Check sheet for the drawn part. Datum: minimum x, y, z corner. Units: mm. A direction names the side the tool comes from. Round coordinates to 2 decimals unless told otherwise and drop trailing zeros. Write each loop counter-clockwise with the first axis right and the second up, starting at its lowest first coordinate (ties: lowest second). Pieces come first, ordered by that corner, then holes. Notation, with made-up numbers: M 54,44.25 L 108,44.25 A7 cw 108,56.25 Z; hole C 13.25,14 d5. An arc over 180 degrees is marked long. One line per item, written item: value. Start each with the question number.
1. Depth check by flat-ended pin: P1, Ø5, axis at x = 35.5, y = 66.5, coming from the +Z side; P2, Ø3, axis at x = 37, y = 32.5, coming from the -Z side; P3, Ø8, axis at x = 83, z = 69, coming from the +Y side. Enter the tip coordinate at first touch or a pass-through.
2. Section check B-B (y = 69.85). Record the boundary of the cut face in (x, z), and give its area (3 significant figures).
3. Section check A-A (x = 50.8). Record the boundary of the cut face in (y, z), and give its area (3 significant figures).
4. Access from +Z, -Z, +X, -X, +Y, -Y to the whole of each face (thin tool, end or side, straight path). Record for the marked faces 1 and 2.
5. Section check D-D (z = 50.8). Record the boundary of the cut face in (x, y).
6. Release check for a two-part mould opening along Z. For the marked faces 3, 4 and 5 record: pulls with the +Z half, pulls with the -Z half, needs draft (parallel to the pull), parting line crosses it, or undercut.
7. Scan lines: probe 1 along Y at (x, z) = (50.8, 92.25); probe 2 along X at (y, z) = (69, 5); probe 3 along X at (y, z) = (69, 97). Record each from-to range of solid material in increasing order. Write a range as [from, to].
8. Section check C-C (y = 57). Record the boundary of the cut face in (x, z).
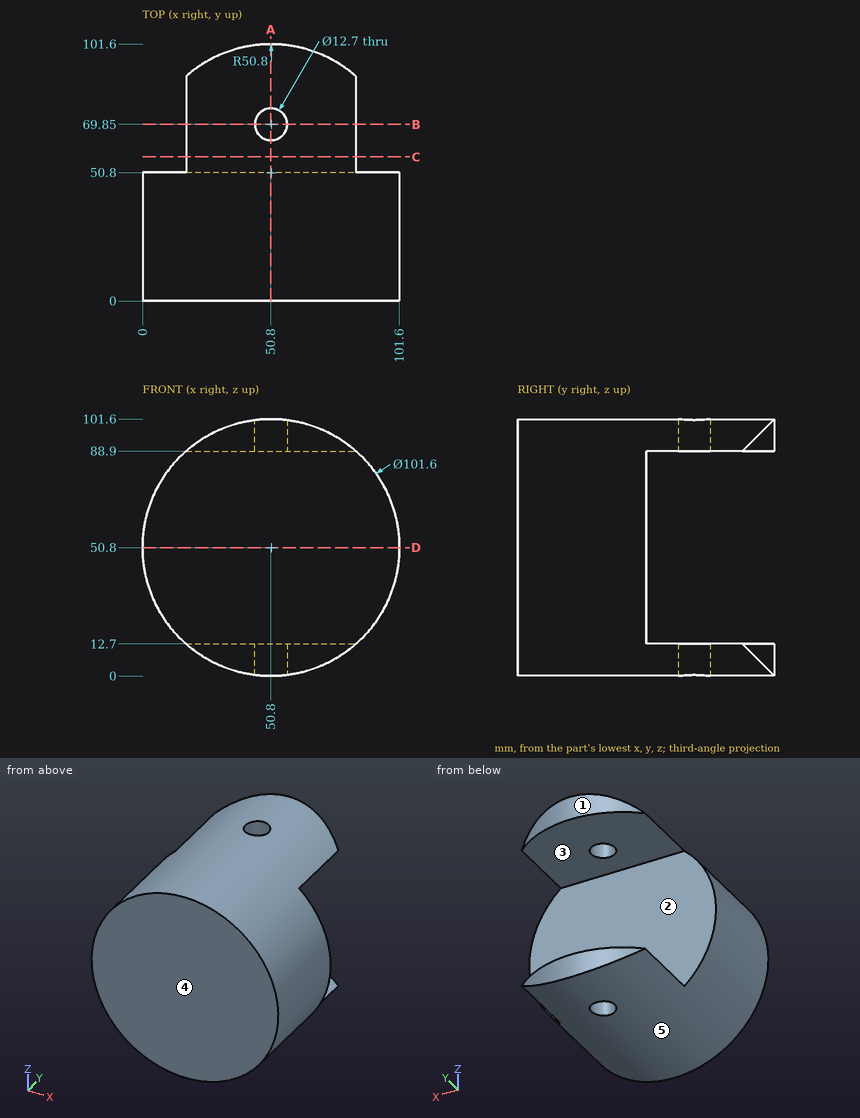
Result sheet:
1. P1: stops at z = 99.96
1. P2: stops at z = 1.51
1. P3: stops at y = 50.8
2. outline: M 17.2,12.7 A50.8 ccw 44.45,0.4 L 44.45,12.7 Z; M 17.2,88.9 L 44.45,88.9 L 44.45,101.2 A50.8 ccw Z; M 57.15,0.4 A50.8 ccw 84.4,12.7 L 57.15,12.7 Z; M 57.15,88.9 L 84.4,88.9 A50.8 ccw 57.15,101.2 Z
2. area: 851 mm2
3. outline: M 0,0 L 63.5,0 L 63.5,12.7 L 50.8,12.7 L 50.8,88.9 L 63.5,88.9 L 63.5,101.6 L 0,101.6 Z; M 76.2,0 L 101.6,0 L 101.6,12.7 L 76.2,12.7 Z; M 76.2,88.9 L 101.6,88.9 L 101.6,101.6 L 76.2,101.6 Z
3. area: 6,130 mm2
4. face 1: +Z, -Z, +Y
4. face 2: +X, -X, +Y
5. outline: M 0,0 L 101.6,0 L 101.6,50.8 L 0,50.8 Z
6. face 3: undercut
6. face 4: needs draft
6. face 5: parting line crosses it
7. probe 1: y = [0, 63.5], [76.2, 101.6]
7. probe 2: x = [28.82, 44.51], [57.09, 72.78]
7. probe 3: x = [29.68, 44.51], [57.09, 71.92]
8. outline: M 17.2,12.7 A50.8 ccw 84.4,12.7 Z; M 17.2,88.9 L 84.4,88.9 A50.8 ccw Z
